from build123d import *

# Parameters (mm, degrees)
SKETCH_1_R          = 1.5
EXTRUDE_1_DEPTH     = 3
CHAMFER_1_SIZE      = 7
FILLET_START        = -1
FILLET_1_DEPTH      = 5
FILLET_1_2_DEPTH    = 3
SKETCH_3_R          = 1.5
SKETCH_3_W          = 40
SKETCH_3_H          = 40
CUT_EXTRUDE_1_DEPTH = 3
FILLET_2_R          = 15


with BuildPart() as part:
    # 草图1 → 凸台-拉伸1 (new body)
    with BuildSketch(Plane(origin=(0, 0, 0), x_dir=(1, 0, 0), z_dir=(0, 1, 0))):
        Polygon((-55, 50), (-55, -50), (55, -50), (55, 50), (43, 50), (43, 105), (-43, 105), (-43, 50), align=None)
        with Locations(Location((-43.343145751, -44, 0), (0, 0, 270))):
            Circle(SKETCH_1_R, mode=Mode.SUBTRACT)
        with Locations(Location((-49, -38.343145751, 0), (0, 0, 270))):
            Circle(SKETCH_1_R, mode=Mode.SUBTRACT)
        with Locations(Location((43.343145751, -44, 0), (0, 0, 270))):
            Circle(SKETCH_1_R, mode=Mode.SUBTRACT)
        with Locations(Location((49, -38.343145751, 0), (0, 0, 270))):
            Circle(SKETCH_1_R, mode=Mode.SUBTRACT)
        with Locations(Location((-49, 38.343145751, 0), (0, 0, 270))):
            Circle(SKETCH_1_R, mode=Mode.SUBTRACT)
        with Locations(Location((-43.343145751, 44, 0), (0, 0, 270))):
            Circle(SKETCH_1_R, mode=Mode.SUBTRACT)
        with Locations(Location((43.343145751, 44, 0), (0, 0, 270))):
            Circle(SKETCH_1_R, mode=Mode.SUBTRACT)
        with Locations(Location((49, 38.343145751, 0), (0, 0, 270))):
            Circle(SKETCH_1_R, mode=Mode.SUBTRACT)
        with Locations(Location((38, 95, 0), (0, 0, 270))):
            Circle(SKETCH_1_R, mode=Mode.SUBTRACT)
        with Locations(Location((-38, 95, 0), (0, 0, 270))):
            Circle(SKETCH_1_R, mode=Mode.SUBTRACT)
    extrude(amount=EXTRUDE_1_DEPTH)

    # 倒角1
    chamfer_1_edges = [part.edges().sort_by_distance(p)[0] for p in [
        (-55, 1.5, 50),
        (-55, 1.5, -50),
        (55, 1.5, -50),
        (55, 1.5, 50),
    ]]
    chamfer(chamfer_1_edges, length=CHAMFER_1_SIZE)

    # 圆角1: read off the stored shape, not the designer's step
    # 圆角1 outline → 圆角1 (cut)
    with BuildSketch(Plane(origin=(0, 0, 0), x_dir=(1, 0, 0), z_dir=(0, 1, 0)).offset(FILLET_START)):
        with BuildLine():
            ThreePointArc((-43, 100), (-41.535533906, 103.535533906), (-38, 105))
            Line((-38, 105), (-43, 105))
            Line((-43, 105), (-43, 100))
        make_face()
        with BuildLine():
            ThreePointArc((38, 105), (41.535533906, 103.535533906), (43, 100))
            Line((43, 100), (43, 105))
            Line((43, 105), (38, 105))
        make_face()
    extrude(amount=FILLET_1_DEPTH, mode=Mode.SUBTRACT)

    # Fillet 1 2 outline → Fillet 1 2 (add)
    with BuildSketch(Plane(origin=(0, 0, 0), x_dir=(1, 0, 0), z_dir=(0, 1, 0))):
        with BuildLine():
            Line((43, 50), (48, 50))
            ThreePointArc((48, 50), (44.464466094, 51.464466094), (43, 55))
            Line((43, 55), (43, 50))
        make_face()
        with BuildLine():
            Line((-43, 50), (-43, 55))
            ThreePointArc((-43, 55), (-44.464466094, 51.464466094), (-48, 50))
            Line((-48, 50), (-43, 50))
        make_face()
    extrude(amount=FILLET_1_2_DEPTH)

    # 草图3 → 切除-拉伸1 (cut)
    with BuildSketch(Plane(origin=(0, 3, 0), x_dir=(1, 0, 0), z_dir=(0, 1, 0))):
        with Locations(Location((-40.14, 29.5, 0), (0, 0, 270))):
            Circle(SKETCH_3_R)
        with Locations(Location((44.86, 27, 0), (0, 0, 270))):
            Circle(SKETCH_3_R)
        with Locations(Location((-38.14, -30, 0), (0, 0, 270))):
            Circle(SKETCH_3_R)
        with Locations(Location((39.86, -30, 0), (0, 0, 270))):
            Circle(SKETCH_3_R)
        Rectangle(SKETCH_3_W, SKETCH_3_H)
    extrude(amount=-CUT_EXTRUDE_1_DEPTH, mode=Mode.SUBTRACT)

    # 圆角2
    fillet_2_edges = [part.edges().sort_by_distance(p)[0] for p in [
        (20, 1.5, -20),
        (20, 1.5, 20),
        (-20, 1.5, 20),
        (-20, 1.5, -20),
    ]]
    fillet(fillet_2_edges, radius=FILLET_2_R)


solid = part.part
Can you work these out from the model? Positions are in its coordinate system, mm. A direction names the side the tool comes from. Round coordinates to 2 decimals unless told otherwise and drop trailing zeros. Write each loop counter-clockwise with the first axis right and the second up, starting at its lowest first coordinate (ties: lowest second). Pieces come first, ordered by that corner, then holes. Notation, with made-up numbers: (2, 53) -> (38, 53) arc R28 cw to (38, 75) -> close; hole circle Ø11 at (-39, 13). An arc over 180 degrees is marked (long way). One line per question, with ' | ' between items. Start each with the question number.
1) Suppose I cut it at C-C on y = 2. Count the separate pieces of the cut face and the enclosed holes in it, then the cut area to 3 significant figures.
2) Suppose I cut it at A-A on z = -3. Write out the boundary of the cut face in (x, y).
3) On a 3-axis mill with a long thin cutter (end or side, diameter ignored), from which of +Z, -Z, +X, -X, +Y, -Y can I reach the whole of each face in a straight line? I mean faces 4 (the flat face through (-51, 1, -47)), 5 (the cylindrical face through (15.49, 1.48, 15.72)). Say none if no direction works.
4) I need wall thicknesses on line 1 (X direction, y = 2.2, z = -27); line 2 (Z direction, x = -4.5, y = 0.4); line 3 (X direction, y = 0.7, z = -44). Which ranges of each line are inside material? Lowest first, please. Write a range as [from, to].
5) Suppose I cut it at B-B on x = -8.5. Write out the boundary of the cut face in (y, z), then the cut area to 3 significant figures.
6) If we mould it in two halves opening along X, with no side actions, what happens to faces 1 (the cylindrical face through (45, 1, -51)), 2 (the flat face through (0, 2, 20)), 3 (the cylindrical face through (-42, 1, -103))? For each: released by +X, released by -X, zero draft, split by the parting line, or undercut.
Return value:
1) separate pieces: 1 | enclosed holes: 15 | area: 14,100 mm2
2) outline: (-55, 0) -> (-20, 0) -> (-20, 3) -> (-55, 3) -> close; (20, 0) -> (55, 0) -> (55, 3) -> (20, 3) -> close
3) face 4: -Z, -X, +Y, -Y | face 5: +Y, -Y
4) line 1: x = [-55, 43.36], [46.36, 55] | line 2: z = [-105, -20], [20, 50] | line 3: x = [-54, -44.84], [-41.84, 41.84], [44.84, 54]
5) outline: (0, -105) -> (3, -105) -> (3, -19.59) -> (0, -19.59) -> close; (0, 19.59) -> (3, 19.59) -> (3, 50) -> (0, 50) -> close | area: 347 mm2
6) face 1: released by +X | face 2: undercut | face 3: released by -X
